```python
from build123d import *

# Parameters (mm, degrees)
SKETCH_1_W      = 100
SKETCH_1_H      = 88
SKETCH_1_R      = 1.25
SKETCH_1_R_2    = 11
EXTRUDE_1_DEPTH = 1.7
FILLET_1_R      = 10


with BuildPart() as part:
    # 草图1 → 凸台-拉伸1 (new body)
    with BuildSketch(Plane.XY):
        Rectangle(SKETCH_1_W, SKETCH_1_H)
        with Locations((-48.25, 23.2)):
            Circle(SKETCH_1_R, mode=Mode.SUBTRACT)
        with Locations((-48.25, -23.2)):
            Circle(SKETCH_1_R, mode=Mode.SUBTRACT)
        with Locations(Location((48.25, -23.2, 0), (0, 0, 180))):
            Circle(SKETCH_1_R, mode=Mode.SUBTRACT)
        with Locations(Location((48.25, 23.2, 0), (0, 0, 180))):
            Circle(SKETCH_1_R, mode=Mode.SUBTRACT)
        Circle(SKETCH_1_R_2, mode=Mode.SUBTRACT)
        with Locations((-28.75, 23.2)):
            Circle(SKETCH_1_R, mode=Mode.SUBTRACT)
        with Locations(Location((-28.75, -23.2, 0), (0, 0, 180))):
            Circle(SKETCH_1_R, mode=Mode.SUBTRACT)
        with Locations((28.75, -23.2)):
            Circle(SKETCH_1_R, mode=Mode.SUBTRACT)
        with Locations(Location((28.75, 23.2, 0), (0, 0, 180))):
            Circle(SKETCH_1_R, mode=Mode.SUBTRACT)
    extrude(amount=EXTRUDE_1_DEPTH)

    # 圆角1
    fillet_1_edges = [part.edges().sort_by_distance(p)[0] for p in [
        (50, -44, 0.85),
        (-50, -44, 0.85),
        (-50, 44, 0.85),
        (50, 44, 0.85),
    ]]
    fillet(fillet_1_edges, radius=FILLET_1_R)


solid = part.part
```
Could you check a few things on this model? Use its own coordinates, in mm. Coordinates: 2 decimals unless noted, no trailing zeros. Loops run counter-clockwise (first coordinate to the right, second up) from the corner with the lowest first, then second, coordinate; pieces in that order, holes last.
1) Imagine slicing it at C-C (z = 0.95). State how many separate pieces and enclosed holes the cut face has, and give its area (3 significant figures).
Reported:
separate pieces: 1
enclosed holes: 9
area: 8,290 mm2
2) Imagine slicing it at D-D (y = -23.2). List the corners of the cut face in (x, z) for me.
Reported:
outline: (-50, 0) - (-49.5, 0) - (-49.5, 1.7) - (-50, 1.7) - close; (-47, 0) - (-30, 0) - (-30, 1.7) - (-47, 1.7) - close; (-27.5, 0) - (27.5, 0) - (27.5, 1.7) - (-27.5, 1.7) - close; (30, 0) - (47, 0) - (47, 1.7) - (30, 1.7) - close; (49.5, 0) - (50, 0) - (50, 1.7) - (49.5, 1.7) - close
3) Please list where these lines run through material, in increasing order: line 1 along X through (y, z) = (-22.5, 0.35); line 2 along Y through (x, z) = (-0.5, 1.15); line 3 along Y through (x, z) = (-48.25, 0.4).
Reported:
line 1: x = -50 to -49.29, -47.21 to -29.79, -27.71 to 27.71, 29.79 to 47.21, 49.29 to 50
line 2: y = -44 to -10.99, 10.99 to 44
line 3: y = -39.65 to -24.45, -21.95 to 21.95, 24.45 to 39.65
4) Imagine slicing it at B-B (y = 0). List the corners of the cut face in (x, z) for me.
Reported:
outline: (-50, 0) - (-11, 0) - (-11, 1.7) - (-50, 1.7) - close; (11, 0) - (50, 0) - (50, 1.7) - (11, 1.7) - close
5) Thinking about a two-plate mould opening in X: for faces 1 (the face through (-47.15, 40.99, 0.86)), 2 (the face through (48.52, 24.42, 0.84)), 3 (the face through (46.99, -41.15, 0.86)), 4 (the face through (-28.078, 24.254, 0.838)), which applies, released by +X, released by -X, zero draft, split by the parting line, or undercut?
Reported:
face 1: released by -X
face 2: undercut
face 3: released by +X
face 4: undercut
6) Imagine slicing it at A-A (x = 0). List the corners of the cut face in (y, z) for me.
Reported:
outline: (-44, 0) - (-11, 0) - (-11, 1.7) - (-44, 1.7) - close; (11, 0) - (44, 0) - (44, 1.7) - (11, 1.7) - close
